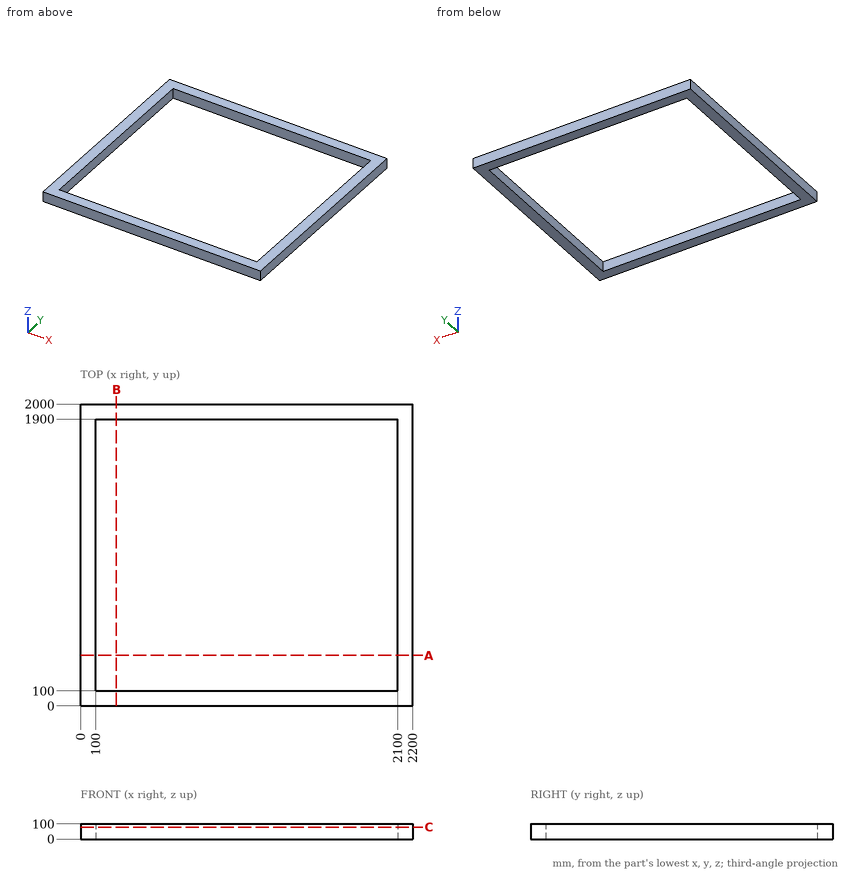
Input: dimensioned drawing with shaded views. Units: mm. Origin: part minimum x, y, z. Give positions to 0.01 mm unless a question says otherwise; leave off trailing zeros. Loops run counter-clockwise (first coordinate to the right, second up) from the corner with the lowest first, then second, coordinate; pieces in that order, holes last. Notation, with made-up numbers: (-35.75, 4) -> (-18.75, 4) arc R18 ccw to (-18.75, 26) -> close; hole circle Ø6 at (74.5, 11). An arc over 180 degrees is marked (long way). Use a Markdown table: item, result. Add a question column.
1) Section query B-B, the plane x = 237.5. Return the cut outline in (y, z).
2) Section query C-C, the plane z = 79. Return the cut outline in (x, y), then the cut area to 3 significant figures.
3) Line query: line 1 along Y through (x, z) = (940, 69.5); line 2 along X through (y, z) = (272, 27.5). Output: solid intervals per line, ascending. Write a range as [from, to].
4) Section query A-A, the plane y = 335. Return the cut outline in (x, z), then the cut area to 3 significant figures.
5) First-contact query: pin 1 (8 mm diameter, centred on y = 289, z = 37, fed in from -X). Flat tip, straight axial feed; report the tip coordinate or a pass-through.
Numbers:
| question | item | result |
|---|---|---|
| 1 | outline | (0, 0) -> (100, 0) -> (100, 100) -> (0, 100) -> close; (1900, 0) -> (2000, 0) -> (2000, 100) -> (1900, 100) -> close |
| 2 | outline | (0, 0) -> (2200, 0) -> (2200, 2000) -> (0, 2000) -> close; hole (100, 100) -> (2100, 100) -> (2100, 1900) -> (100, 1900) -> close |
| 2 | area | 800,000 mm2 |
| 3 | line 1 | y = [0, 100], [1900, 2000] |
| 3 | line 2 | x = [0, 100], [2100, 2200] |
| 4 | outline | (0, 0) -> (100, 0) -> (100, 100) -> (0, 100) -> close; (2100, 0) -> (2200, 0) -> (2200, 100) -> (2100, 100) -> close |
| 4 | area | 20,000 mm2 |
| 5 | pin 1 | stops at x = 0 |
